For this review, take the finished solid that the model builds, in its own axes (mm). Round coordinates to 2 decimals unless told otherwise and drop trailing zeros. Loops run counter-clockwise (first coordinate to the right, second up) from the corner with the lowest first, then second, coordinate; pieces in that order, holes last. Notation, with made-up numbers: M -25,1.25 L 19,1.25 A16 cw 19,30.25 Z; hole C 16,25.5 d10. An arc over 180 degrees is marked long. One line per question, with ' | ' between items. Start each with the question number.
1) We need section A-A (x = 0). Give the boundary of the cut face in (y, z), and give its area (3 significant figures).
2) We need section B-B (z = 0). Give the boundary of the cut face in (x, y).
3) We need section C-C (y = -0.75). Give the boundary of the cut face in (x, z), and give its area (3 significant figures).
4) For pin 1 Ø3 at (y, z) = (7.5, -2) entering from -X; pin 2 Ø1.6 at (x, z) = (1.5, -0.5) entering from -Y, all flat-tipped, find the tip position at first contact; note any pin that passes through.
5) We need section D-D (y = 7). Give the boundary of the cut face in (x, z), and give its area (3 significant figures).
6) For probe 1 along Y at (x, z) = (-0.25, 2.6); probe 2 along X at (y, z) = (4.5, -0.1); probe 3 along X at (y, z) = (3, 0.85), list the stretches that pass through material, from the lowest coordinate up. Write a range as from..to.
Autodesk Inventor part; units mm, degrees
ref_plane "YZ Plane" through (0, 0, 0) normal (1, 0, 0) x (0, 1, 0)
ref_plane "XZ Plane" through (0, 0, 0) normal (0, 1, 0) x (-1, 0, 0)
ref_plane "XY Plane" through (0, 0, 0) normal (0, 0, 1) x (1, 0, 0)
sketch "スケッチ1" plane through (0, 0, 0) normal (0, 1, 0) x (-1, 0, 0)
  circle A0 centre (0, 0) radius 3
  dimension "d0" = 6
extrude "押し出し1" add sketch "スケッチ1" along normal blind 12
chamfer "面取り1" distance 0.3 angle 45 1 edges at (3, 0, 0)
sketch "スケッチ2" plane through (0, 0, 0) normal (0, -1, 0) x (1, 0, 0)
  circle A0 centre (0, 0) radius 0.4
  dimension "d6" = 0.8
extrude "押し出し2" add sketch "スケッチ2" along normal blind 3.5
properties part number "FanMotor"
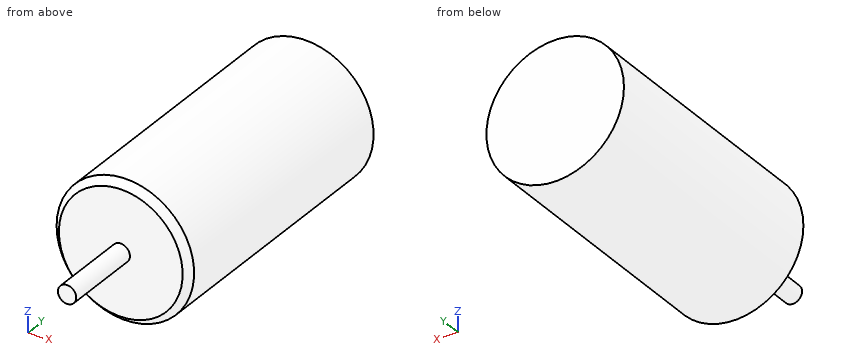
Answers below:
1) outline: M -3.5,-0.4 L 0,-0.4 L 0,-2.7 L 0.3,-3 L 12,-3 L 12,3 L 0.3,3 L 0,2.7 L 0,0.4 L -3.5,0.4 Z | area: 74.7 mm^2
2) outline: M -3,0.3 L -2.7,0 L -0.4,0 L -0.4,-3.5 L 0.4,-3.5 L 0.4,0 L 2.7,0 L 3,0.3 L 3,12 L -3,12 Z
3) outline: C 0,0 d0.8 | area: 0.503 mm^2
4) pin 1: x = -2.96 | pin 2: y = 0
5) outline: C 0,0 d6 | area: 28.3 mm^2
6) probe 1: 0..12 | probe 2: -3..3 | probe 3: -2.88..2.88
